For this review, take the finished solid that the model builds, in its own axes (mm). Face numbers are marked on the shaded views. A direction names the side the tool comes from. Coordinates: 2 decimals unless noted, no trailing zeros. Order: outer loops, then holes, each group sorted by start corner. A loop starts at its lowest first (then second) coordinate and runs counter-clockwise, first axis right, second up. Notation, with made-up numbers: M 31.25,39.25 L 40.25,39.25 A15 cw 40.25,57.25 Z; hole C 62.25,49.25 d2. An arc over 180 degrees is marked long. Use one line per item in the form item = value. Start each with the question number.
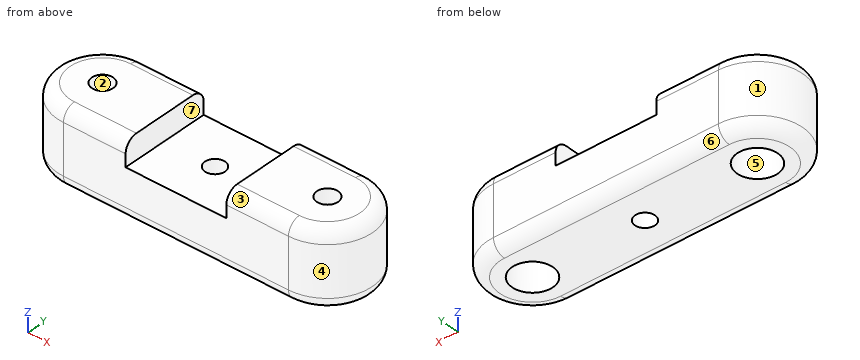
```python
from build123d import *

# Parameters (mm, degrees)
BOSS_EXTRUDE1_START = 1220
SKETCH1_R           = 8.1
BOSS_EXTRUDE1_DEPTH = 30
SKETCH3_R           = 8.1
SKETCH3_R_2         = 4.25
BOSS_EXTRUDE2_DEPTH = 10
SKETCH4_W           = 40.3
SKETCH4_H           = 36
CUT_EXTRUDE1_DEPTH  = 10
FILLET1_R           = 5
FILLET2_R           = 5
SKETCH5_R           = 4
CUT_EXTRUDE2_DEPTH  = 50


with BuildPart() as part:
    # Sketch1 → Boss-Extrude1 (new body)
    with BuildSketch(Plane.XY.offset(BOSS_EXTRUDE1_START)):
        with BuildLine():
            Line((-45, 18), (45, 18))
            ThreePointArc((45, 18), (63, 0), (45, -18))
            Line((45, -18), (-45, -18))
            ThreePointArc((-45, -18), (-63, 0), (-45, 18))
        make_face()
        with Locations((-45, 0)):
            Circle(SKETCH1_R, mode=Mode.SUBTRACT)
        with Locations((45, 0)):
            Circle(SKETCH1_R, mode=Mode.SUBTRACT)
    extrude(amount=-BOSS_EXTRUDE1_DEPTH)

    # Sketch3 → Boss-Extrude2 (add)
    # profile 1 of 2: a face of its own
    with BuildSketch(Plane.XY.offset(1220)):
        with Locations((45, 0)):
            Circle(SKETCH3_R)
        with Locations((45, 0)):
            Circle(SKETCH3_R_2, mode=Mode.SUBTRACT)
    # profile 2 of 2: a face of its own
    with BuildSketch(Plane.XY.offset(1220)):
        with Locations((-45, 0)):
            Circle(SKETCH3_R)
        with Locations((-45, 0)):
            Circle(SKETCH3_R_2, mode=Mode.SUBTRACT)
    extrude(amount=-BOSS_EXTRUDE2_DEPTH)

    # Sketch4 → Cut-Extrude1 (cut)
    with BuildSketch(Plane.XY.offset(1220)):
        Rectangle(SKETCH4_W, SKETCH4_H)
    extrude(amount=-CUT_EXTRUDE1_DEPTH, mode=Mode.SUBTRACT)

    # Fillet1
    fillet1_edges = [part.edges().sort_by_distance(p)[0] for p in [
        (63, 0, 1190),
        (0, 18, 1190),
        (-63, 0, 1190),
        (0, -18, 1190),
    ]]
    fillet(fillet1_edges, radius=FILLET1_R)

    # Fillet2
    fillet2_edges = [part.edges().sort_by_distance(p)[0] for p in [
        (32.575, -18, 1220),
        (-32.575, 18, 1220),
        (32.575, 18, 1220),
        (63, 0, 1220),
        (-32.575, -18, 1220),
        (-63, 0, 1220),
    ]]
    fillet(fillet2_edges, radius=FILLET2_R)

    # Sketch5 → Cut-Extrude2 (cut)
    with BuildSketch(Plane.XY.offset(1210)):
        Circle(SKETCH5_R)
    extrude(amount=-CUT_EXTRUDE2_DEPTH, mode=Mode.SUBTRACT)


solid = part.part
```
1. The part is to be moulded in two halves that separate along X. For the marked faces 1, 2, 3 and 4, say which applies: pulls with the +X half, pulls with the -X half, needs draft (parallel to the pull), parting line crosses it, or undercut.
2. Consider section C-C, the plane y = 0. Give the number of separate pieces and of enclosed holes in the cut face, plus the area to 3 significant figures.
3. Consider section A-A, the plane x = 0. Write out the cut boundary in (y, z), plus the area to 3 significant figures.
4. Consider section B-B, the plane z = 1212.5. Write out the cut boundary in (x, y), plus the area to 3 significant figures.
5. Tool access review of the marked faces 5, 6 and 7: name each direction out of +Z, -Z, +X, -X, +Y, -Y from which nothing blocks a thin tool from reaching the whole face with its end or side.
6. Consider section D-D, the plane z = 1196.5. Write out the cut boundary in (x, y).
7. For pin 1 Ø13 at (x, y) = (-45, 0) entering from -Z; pin 2 Ø4 at (y, z) = (-7.5, 1214.5) entering from -X; pin 3 Ø1 at (y, z) = (3.5, 1204) entering from -X, all flat-tipped, find the tip position at first contact; note any pin that passes through.
8. To check wall thickness, follow line 1 (Y direction, x = -45, z = 1197); line 2 (Z direction, x = -13, y = 0); line 3 (X direction, y = 12.5, z = 1218). State the ranges of each line that lie inside material, in increasing order.
Answers follow:
q1.face_1 = pulls with the -X half
q1.face_2 = undercut
q1.face_3 = needs draft
q1.face_4 = pulls with the +X half
q2.separate_pieces = 4
q2.enclosed_holes = 0
q2.area = 2,380 mm²
q3.outline = M -18,1195 A5 ccw -13,1190 L -4,1190 L -4,1210 L -18,1210 Z; M 4,1190 L 13,1190 A5 ccw 18,1195 L 18,1210 L 4,1210 Z
q3.area = 549 mm²
q4.outline = M -45,-18 L -20.15,-18 L -20.15,18 L -45,18 A18 ccw Z; M 20.15,-18 L 45,-18 A18 ccw 45,18 L 20.15,18 Z; hole C -45,0 d8.5; hole C 45,0 d8.5
q4.area = 2,690 mm²
q5.face_5 = -Z
q5.face_6 = -Z, +X, -X, +Y
q5.face_7 = +Z, +Y, -Y
q6.outline = M -45,-18 L 45,-18 A18 ccw 45,18 L -45,18 A18 ccw Z; hole C -45,0 d16.2; hole C 0,0 d8; hole C 45,0 d16.2
q7.pin_1 = 1210
q7.pin_2 = -62.14
q7.pin_3 = -62.75
q8.line_1 = -18 to -8.1, 8.1 to 18
q8.line_2 = 1190 to 1210
q8.line_3 = -56.52 to -20.15, 20.15 to 56.52
